from build123d import *

# Parameters (mm, degrees)
SKETCH1_R           = 1.7
BOSS_EXTRUDE1_DEPTH = 3.5
SKETCH2_R           = 12.1
SKETCH2_R_2         = 9.6
BOSS_EXTRUDE2_DEPTH = 7
SKETCH3_W           = 47.11
SKETCH3_H           = 55
BOSS_EXTRUDE3_DEPTH = 3.5
SKETCH4_R           = 1.7
CUT_EXTRUDE1_DEPTH  = 89.787375369
SKETCH5_W           = 5.655
SKETCH5_H           = 25
CUT_EXTRUDE2_DEPTH  = 77.768795907
FILLET3_R           = 3
FILLET4_R           = 8


with BuildPart() as part:
    # Sketch1 → Boss-Extrude1 (new body)
    with BuildSketch(Plane(origin=(0, 0, 0), x_dir=(1, 0, 0), z_dir=(0, 1, 0))):
        Polygon((-23.555, 17.5), (-23.555, -17.5), (23.555, -17.5), (23.555, 17.5), (23.555, 44.6), (-23.555, 44.6), align=None)
        with Locations(Location((-18.555, -12.5, 0), (0, 0, 270))):
            Circle(SKETCH1_R, mode=Mode.SUBTRACT)
        with Locations(Location((-18.555, 12.5, 0), (0, 0, 90))):
            Circle(SKETCH1_R, mode=Mode.SUBTRACT)
        with Locations(Location((18.555, -12.5, 0), (0, 0, 90))):
            Circle(SKETCH1_R, mode=Mode.SUBTRACT)
        with Locations(Location((18.555, 12.5, 0), (0, 0, 270))):
            Circle(SKETCH1_R, mode=Mode.SUBTRACT)
    extrude(amount=BOSS_EXTRUDE1_DEPTH)

    # Sketch2 → Boss-Extrude2 (add)
    with BuildSketch(Plane(origin=(0, 3.5, 0), x_dir=(1, 0, 0), z_dir=(0, 1, 0))):
        with Locations(Location((0, 0, 0), (0, 0, 90))):
            Circle(SKETCH2_R)
        with Locations(Location((0, 0, 0), (0, 0, 270))):
            Circle(SKETCH2_R_2, mode=Mode.SUBTRACT)
    extrude(amount=BOSS_EXTRUDE2_DEPTH)

    # Sketch3 → Boss-Extrude3 (add)
    with BuildSketch(Plane(origin=(0, 0, -44.6), x_dir=(-1, 0, 0), z_dir=(0, 0, -1))):
        with Locations((0, 27.5)):
            Rectangle(SKETCH3_W, SKETCH3_H)
    extrude(amount=BOSS_EXTRUDE3_DEPTH)

    # Sketch4 → Cut-Extrude1 (cut, through all)
    with BuildSketch(Plane(origin=(0, 0, -48.1), x_dir=(-1, 0, 0), z_dir=(0, 0, -1))):
        with Locations((-10, 47.5)):
            Circle(SKETCH4_R)
        with Locations((-10, 27.5)):
            Circle(SKETCH4_R)
        with Locations((10, 27.5)):
            Circle(SKETCH4_R)
        with Locations((10, 47.5)):
            Circle(SKETCH4_R)
    extrude(amount=-CUT_EXTRUDE1_DEPTH, mode=Mode.SUBTRACT)

    # Sketch5 → Cut-Extrude2 (cut, through all)
    with BuildSketch(Plane(origin=(0, 55, 0), x_dir=(1, 0, 0), z_dir=(0, 1, 0))):
        with Locations((-20.7275, 35.6)):
            Rectangle(SKETCH5_W, SKETCH5_H)
        with Locations((20.7275, 35.6)):
            Rectangle(SKETCH5_W, SKETCH5_H)
    extrude(amount=-CUT_EXTRUDE2_DEPTH, mode=Mode.SUBTRACT)

    # Fillet3
    fillet3_edges = [part.edges().sort_by_distance(p)[0] for p in [
        (23.555, 1.75, -23.1),
        (23.555, 1.75, 17.5),
        (-23.555, 1.75, 17.5),
        (-23.555, 1.75, -23.1),
    ]]
    fillet(fillet3_edges, radius=FILLET3_R)

    # Fillet4
    fillet4_edges = [part.edges().sort_by_distance(p)[0] for p in [
        (0, 3.5, -44.6),
    ]]
    fillet(fillet4_edges, radius=FILLET4_R)


solid = part.part
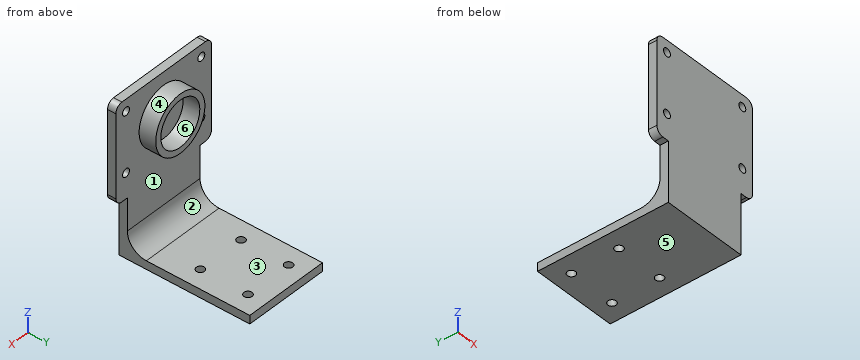
Part model, mm, in its own coordinate system. Face numbers are marked on the shaded views. A direction names the side the tool comes from. Coordinates: 2 decimals unless noted, no trailing zeros. Loops run counter-clockwise (first coordinate to the right, second up) from the corner with the lowest first, then second, coordinate; pieces in that order, holes last. Notation, with made-up numbers: (71, -34) -> (84, -34) arc R33 ccw to (84, 4) -> close; hole circle Ø1 at (80, -34.75). An arc over 180 degrees is marked (long way). Use a Markdown table: item, result. Add a question column.
Item 1: Pull direction X, two halves, no side cores. Call the marked faces 4, 5 and 6: +X half, -X half, draft (parallel to the pull), parting line (faces both ways), or undercut.
Item 2: Flat gauge pins, fed straight in: P1, Ø8, axis at x = -10.5, y = 42, coming from the +Z side; P2, Ø7.5, axis at x = 2, z = -4, coming from the +Y side; P3, Ø3, axis at x = 18.555, z = 12.5, coming from the -Y side; P4, Ø10, axis at x = 7.5, y = 12.5, coming from the +Z side. Where does each tip first touch, or does it go through?
Item 3: Probe probe 1 along Y at (x, z) = (10, -46.1); probe 2 along X at (y, z) = (2.55, -12.5) (3 decimals); probe 3 along X at (y, z) = (7.25, 0). List the from-to ranges inside material, lowest first.
Item 4: Band-saw the part on C-C on z = -1.5. Write the cut outline in (x, y) (3 decimals), plus the area to 3 significant figures.
Item 5: Which spindle directions (+Z, -Z, +X, -X, +Y, -Y) get a long thin tool onto all of the face, cutting with end or side? Do the marked faces 1, 2 and 3. Say none if no direction does.
Item 6: Band-saw the part on D-D on y = 37.5. Write the cut outline in (x, z), plus the area to 3 significant figures.
Item 7: Band-saw the part on B-B on x = 16. Write the cut outline in (y, z), plus the area to 3 significant figures.
Item 8: Band-saw the part on A-A on y = 27.5. Write the cut outline in (x, z).
Geometry says:
| question | item | result |
|---|---|---|
| 1 | face 4 | parting line |
| 1 | face 5 | draft |
| 1 | face 6 | undercut |
| 2 | P1 | z = -44.6 |
| 2 | P2 | y = 3.5 |
| 2 | P3 | through |
| 2 | P4 | z = 11.74 |
| 3 | probe 1 | 0 to 25.8, 29.2 to 45.8, 49.2 to 55 |
| 3 | probe 2 | -23.555 to -20.255, -16.855 to 16.855, 20.255 to 23.555 |
| 3 | probe 3 | -12.1 to -9.6, 9.6 to 12.1 |
| 4 | outline | (-23.555, 0) -> (23.555, 0) -> (23.555, 3.5) -> (12.007, 3.5) -> (12.007, 10.5) -> (9.482, 10.5) -> (9.482, 3.5) -> (-9.482, 3.5) -> (-9.482, 10.5) -> (-12.007, 10.5) -> (-12.007, 3.5) -> (-23.555, 3.5) -> close |
| 4 | area | 200 mm² |
| 5 | face 1 | +Y |
| 5 | face 2 | +X, -X, +Y |
| 5 | face 3 | +Z, +X, -X, +Y |
| 6 | outline | (-17.9, -48.1) -> (17.9, -48.1) -> (17.9, -44.6) -> (-17.9, -44.6) -> close |
| 6 | area | 125 mm² |
| 7 | outline | (0, -48.1) -> (55, -48.1) -> (55, -44.6) -> (11.5, -44.6) arc R8 cw to (3.5, -36.6) -> (3.5, 17.5) -> (0, 17.5) -> close |
| 7 | area | 424 mm² |
| 8 | outline | (-17.9, -48.1) -> (-11.7, -48.1) -> (-11.7, -44.6) -> (-17.9, -44.6) -> close; (-8.3, -48.1) -> (8.3, -48.1) -> (8.3, -44.6) -> (-8.3, -44.6) -> close; (11.7, -48.1) -> (17.9, -48.1) -> (17.9, -44.6) -> (11.7, -44.6) -> close |
